Input: dimensioned drawing with shaded views. Units: mm. Origin: part minimum x, y, z. A direction names the side the tool comes from. Give positions to 0.01 mm unless a question says otherwise; leave off trailing zeros. Write each loop counter-clockwise with the first axis right and the second up, starting at its lowest first coordinate (ties: lowest second). Pieces come first, ordered by that corner, then holes. Notation, with made-up numbers: (-9, 42) -> (4, 42) arc R17 cw to (4, 66) -> close; hole circle Ø7 at (-36, 14.5). An arc over 180 degrees is marked (long way). Answer as a JSON object with one key per item and string values. Group by question number.
(1) Contact query for flat-ended pins moving along their axis: pin 1 Ø1 at (x, z) = (4.5, 0.5) entering from -Y; pin 2 Ø0.9 at (y, z) = (31.5, 2) entering from +X; pin 3 Ø0.6 at (x, z) = (19.5, 2) entering from -Y. Output: stop coordinate, or through.
(2) Section query A-A on x = 19.5. Output: boundary loops of the cut face in (y, z).
(3) Set-up query: the marked faces 1, 2 and 3. Return all of +Z, -Z, +X, -X, +Y, -Y with unobstructed straight access to the full face (end or side cutting, diameter ignored); none if empty.
(4) Section query C-C on y = 21. Output: boundary loops of the cut face in (x, z), plus the area to 3 significant figures.
(5) Section query B-B on x = 36.5. Output: boundary loops of the cut face in (y, z), plus the area to 3 significant figures.
(6) Material intervals for probe 1 along Y at (x, z) = (36.5, 0.7); probe 2 along Y at (x, z) = (6.5, 0.85); probe 3 along X at (y, z) = (4.5, 2.6), sorted ascending.
(7) Section query D-D on x = 6.5. Output: boundary loops of the cut face in (y, z).
(8) Draft query along X for the marked faces 4, 5, 6 and 7. Return one class per face: +X half, -X half, draft (parallel to the pull), parting line (faces both ways), or undercut.
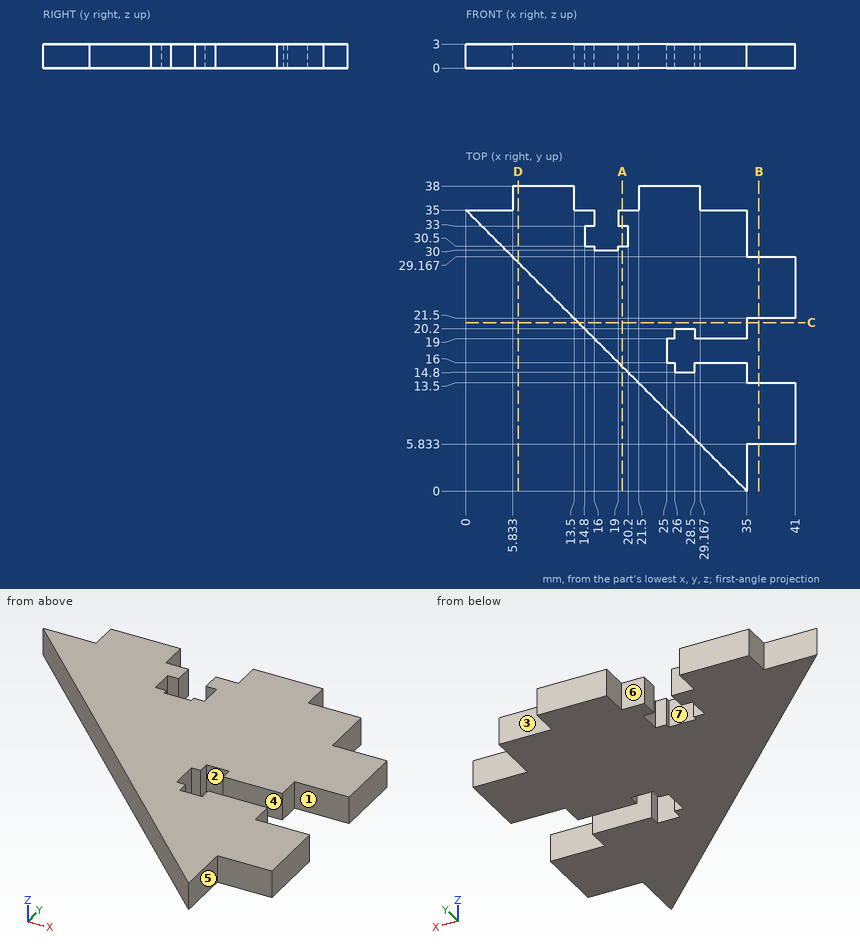
Answer list:
{
 "1": {"pin 1": "y = 30", "pin 2": "x = 35", "pin 3": "y = 15.2"},
 "2": {"outline": "(15.5, 0) -> (30.5, 0) -> (30.5, 3) -> (15.5, 3) -> close; (33, 0) -> (35, 0) -> (35, 3) -> (33, 3) -> close"},
 "3": {"face 1": "+Z, -Z, +X", "face 2": "+Z, -Z", "face 3": "+Z, -Z, +X, +Y"},
 "4": {"outline": "(14, 0) -> (35, 0) -> (35, 3) -> (14, 3) -> close", "area": "63.0 mm2"},
 "5": {"outline": "(5.83, 0) -> (13.5, 0) -> (13.5, 3) -> (5.83, 3) -> close; (21.5, 0) -> (29.17, 0) -> (29.17, 3) -> (21.5, 3) -> close", "area": "46.0 mm2"},
 "6": {"probe 1": "5.83 to 13.5, 21.5 to 29.17", "probe 2": "28.5 to 38", "probe 3": "30.5 to 35"},
 "7": {"outline": "(28.5, 0) -> (38, 0) -> (38, 3) -> (28.5, 3) -> close"},
 "8": {"face 4": "draft", "face 5": "+X half", "face 6": "undercut", "face 7": "undercut"}
}
